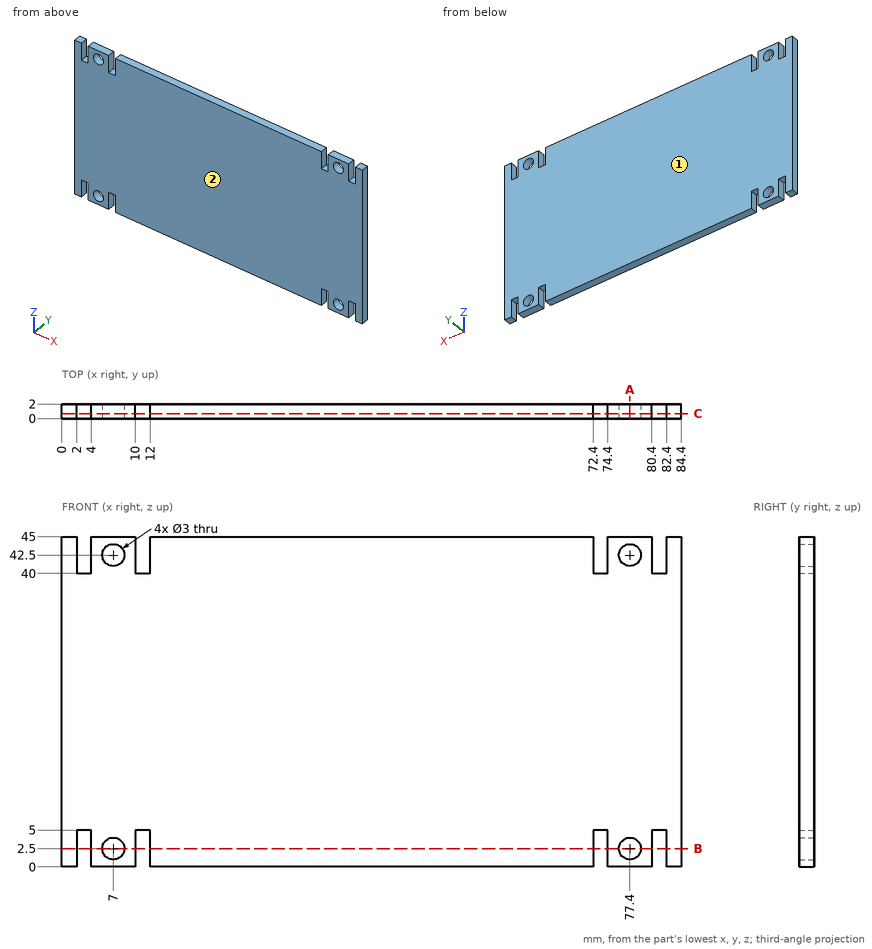
Could you check a few things on this drawing? It's one solid part, dimensions in mm from its lowest x, y, z. Coordinates: 2 decimals unless noted, no trailing zeros. Write each loop counter-clockwise with the first axis right and the second up, starting at its lowest first coordinate (ties: lowest second). Pieces come first, ordered by that corner, then holes.
Q1. Imagine slicing it at C-C, the plane y = 0.7. Count the separate pieces of the cut face and the enclosed holes in it, plus the area to 3 significant figures.
Results found:
separate pieces: 1
enclosed holes: 4
area: 3,690 mm2
Q2. Imagine slicing it at A-A, the plane x = 77.4. List the corners of the cut face in (y, z) for me.
Results found:
outline: (0, 0) - (2, 0) - (2, 1) - (0, 1) - close; (0, 4) - (2, 4) - (2, 41) - (0, 41) - close; (0, 44) - (2, 44) - (2, 45) - (0, 45) - close
Q3. Imagine slicing it at B-B, the plane z = 2.5. List the corners of the cut face in (x, y) for me.
Results found:
outline: (0, 0) - (2, 0) - (2, 2) - (0, 2) - close; (4, 0) - (5.5, 0) - (5.5, 2) - (4, 2) - close; (8.5, 0) - (10, 0) - (10, 2) - (8.5, 2) - close; (12, 0) - (72.4, 0) - (72.4, 2) - (12, 2) - close; (74.4, 0) - (75.9, 0) - (75.9, 2) - (74.4, 2) - close; (78.9, 0) - (80.4, 0) - (80.4, 2) - (78.9, 2) - close; (82.4, 0) - (84.4, 0) - (84.4, 2) - (82.4, 2) - close
Q4. If we mould it in two halves opening along Y, with no side actions, what happens to the marked faces 1 and 2? For each: +Y half, -Y half, draft (parallel to the pull), parting line (faces both ways), or undercut.
Results found:
face 1: +Y half
face 2: -Y half
Q5. For P1, Ø0.6, axis at x = 3.5, y = 0.5, coming from the +Z side, with a flat end and sliding along its axis, tell me the tip position at first contact or that it passes through.
Results found:
P1: stops at z = 40
Q6. Please list where these lines run through material, in increasing order: L1, parallel to Z at x = 8, y = 1.4; L2, parallel to Z at x = 78, y = 0.35.
Results found:
L1: z = 0 to 1.38, 3.62 to 41.38, 43.62 to 45
L2: z = 0 to 1.13, 3.87 to 41.13, 43.87 to 45
